Could you check a few things on this model? Use its own coordinates, in mm. A direction names the side the tool comes from. Give positions to 0.01 mm unless a question says otherwise; leave off trailing zeros. Loops run counter-clockwise (first coordinate to the right, second up) from the corner with the lowest first, then second, coordinate; pieces in that order, holes last.
1. Imagine slicing it at A-A (x = 23). List the corners of the cut face in (y, z) for me, plus the area to 3 significant figures.
2. Thinking about a two-plate mould opening in Y: for faces 3 (the flat face through (-30, -50, 2)), 4 (the flat face through (-37.5, -1, 2)), 5 (the flat face through (-3, 57.5, 2)), which applies, +Y half, -Y half, draft (parallel to the pull), parting line (faces both ways), or undercut?
3. Imagine slicing it at B-B (z = 2.2). Count the separate pieces of the cut face and the enclosed holes in it, plus the area to 3 significant figures.
4. I need wall thicknesses on line 1 along Y through (x, z) = (-20, 3.3); line 2 along X through (y, z) = (-49.5, 1.25). Which ranges of each line are inside material? Lowest first, please.
5. For faces 1 (the flat face through (-1, 1, 4.5)), 2 (the flat face through (22, 32.5, 2)), which set-ups out of +Z, -Z, +X, -X, +Y, -Y let a thin tool reach every point of the face, with its end or its side?
```python
from build123d import *

# Parameters (mm, degrees)
SKETCH1_W           = 75
SKETCH1_H           = 115
SKETCH1_W_2         = 15
SKETCH1_H_2         = 4.5
BOSS_EXTRUDE1_DEPTH = 4.5
FILLET1_R           = 5


with BuildPart() as part:
    # Sketch1 → Boss-Extrude1 (new body)
    with BuildSketch(Plane.XY):
        Rectangle(SKETCH1_W, SKETCH1_H)
        with Locations((22.5, 34.75)):
            Rectangle(SKETCH1_W_2, SKETCH1_H_2, mode=Mode.SUBTRACT)
        with Locations((-22.5, 34.75)):
            Rectangle(SKETCH1_W_2, SKETCH1_H_2, mode=Mode.SUBTRACT)
        with Locations((22.5, -10)):
            Rectangle(SKETCH1_W_2, SKETCH1_H_2, mode=Mode.SUBTRACT)
        with Locations((-22.5, -10)):
            Rectangle(SKETCH1_W_2, SKETCH1_H_2, mode=Mode.SUBTRACT)
        with Locations((22.5, -49.5)):
            Rectangle(SKETCH1_W_2, SKETCH1_H_2, mode=Mode.SUBTRACT)
        with Locations((-22.5, -49.5)):
            Rectangle(SKETCH1_W_2, SKETCH1_H_2, mode=Mode.SUBTRACT)
    extrude(amount=BOSS_EXTRUDE1_DEPTH)

    # Fillet1
    fillet1_edges = [part.edges().sort_by_distance(p)[0] for p in [
        (37.5, 57.5, 2.25),
    ]]
    fillet(fillet1_edges, radius=FILLET1_R)


solid = part.part
```
Derived:
1. outline: (-57.5, 0) - (-51.75, 0) - (-51.75, 4.5) - (-57.5, 4.5) - close; (-47.25, 0) - (-12.25, 0) - (-12.25, 4.5) - (-47.25, 4.5) - close; (-7.75, 0) - (32.5, 0) - (32.5, 4.5) - (-7.75, 4.5) - close; (37, 0) - (57.5, 0) - (57.5, 4.5) - (37, 4.5) - close
1. area: 457 mm2
2. face 3: undercut
2. face 4: draft
2. face 5: +Y half
3. separate pieces: 1
3. enclosed holes: 6
3. area: 8,210 mm2
4. line 1: y = -57.5 to -51.75, -47.25 to -12.25, -7.75 to 32.5, 37 to 57.5
4. line 2: x = -37.5 to -30, -15 to 15, 30 to 37.5
5. face 1: +Z, +X, -X, +Y, -Y
5. face 2: +Z, -Z
